from build123d import *

# Parameters (mm, degrees)
SKETCH1_R               = 4.765
BOSS_EXTRUDE2_DEPTH     = 9.5
CHAMFER1_SIZE           = 2.54
CHAMFER1_SIZE2          = 7.62
CHAMFER1_PART_2_SIZE    = 2.54
CHAMFER1_PART_2_SIZE2   = 7.62
CHAMFER2_SIZE           = 7.62
CHAMFER2_SIZE2          = 2.54
SKETCH3_W               = 9.53
SKETCH3_H               = 9.53
CUT_EXTRUDE1_DEPTH      = 20.54
CUT_EXTRUDE2_DEPTH      = 10.77
CUT_EXTRUDE2_DEPTH_BACK = 10.77
SKETCH5_R               = 1.59
CUT_EXTRUDE3_DEPTH      = 10.5000001
CUT_EXTRUDE3_DEPTH_BACK = 10.5000001


with BuildPart() as part:
    # Sketch1 → Boss-Extrude2 (new body, symmetric)
    with BuildSketch(Plane.XY):
        with BuildLine():
            Line((0, 9.77), (-22.23, 9.77))
            Line((-22.23, 9.77), (-22.23, 4.77))
            Line((-22.23, 4.77), (-9.711509246, -1.067468107))
            ThreePointArc((-9.711509246, -1.067468107), (-6.021421721, -7.693853421), (1.29754109, -9.683454297))
            Line((1.29754109, -9.683454297), (28.58, -6.027722532))
            Line((28.58, -6.027722532), (28.58, 0))
            Line((28.58, 0), (9.77, 0))
            ThreePointArc((9.77, 0), (6.908433252, 6.908433252), (0, 9.77))
        make_face()
        Circle(SKETCH1_R, mode=Mode.SUBTRACT)
    extrude(amount=BOSS_EXTRUDE2_DEPTH, both=True)

    # Chamfer1
    chamfer1_edges = [part.edges().sort_by_distance(p)[0] for p in [
        (-22.23, 7.27, 9.5),
    ]]
    chamfer1_side = [part.faces().sort_by_distance(p)[0] for p in [
        (-22.23, 7.27, 0),
    ]]
    chamfer(chamfer1_edges, length=CHAMFER1_SIZE, length2=CHAMFER1_SIZE2, reference=chamfer1_side[0])

    # Chamfer1 part 2
    chamfer1_part_2_edges = [part.edges().sort_by_distance(p)[0] for p in [
        (28.58, -3.013861266, 9.5),
    ]]
    chamfer1_part_2_side = [part.faces().sort_by_distance(p)[0] for p in [
        (28.58, -3.013861266, 0),
    ]]
    chamfer(chamfer1_part_2_edges, length=CHAMFER1_PART_2_SIZE, length2=CHAMFER1_PART_2_SIZE2, reference=chamfer1_part_2_side[0])

    # Chamfer2
    chamfer2_edges = [part.edges().sort_by_distance(p)[0] for p in [
        (-22.23, 7.27, -9.5),
        (28.58, -3.013861266, -9.5),
    ]]
    chamfer2_side = [part.faces().sort_by_distance(p)[0] for p in [
        (-11.115, 9.225622585, -9.5),
    ]]
    chamfer(chamfer2_edges, length=CHAMFER2_SIZE, length2=CHAMFER2_SIZE2, reference=chamfer2_side[0])

    # Sketch3 → Cut-Extrude1 (cut, through all)
    with BuildSketch(Plane(origin=(0, 9.77, 0), x_dir=(1, 0, 0), z_dir=(0, 1, 0))):
        with Locations((-17.465, 0)):
            Rectangle(SKETCH3_W, SKETCH3_H)
        with Locations((23.815, 0)):
            Rectangle(SKETCH3_W, SKETCH3_H)
    extrude(amount=-CUT_EXTRUDE1_DEPTH, mode=Mode.SUBTRACT)

    # Sketch4 → Cut-Extrude2 (cut, two sides)
    with BuildSketch(Plane(origin=(0, 0, 0), x_dir=(1, 0, 0), z_dir=(0, 1, 0))) as cut_extrude2_sk:
        with BuildLine():
            Line((-3.81, 5.08), (6.35, 5.08))
            ThreePointArc((6.35, 5.08), (11.43, 0), (6.35, -5.08))
            Line((6.35, -5.08), (-3.81, -5.08))
            ThreePointArc((-3.81, -5.08), (-8.89, 0), (-3.81, 5.08))
        make_face()
    extrude(amount=CUT_EXTRUDE2_DEPTH, mode=Mode.SUBTRACT)
    extrude(cut_extrude2_sk.sketch, amount=-CUT_EXTRUDE2_DEPTH_BACK, mode=Mode.SUBTRACT)

    # Sketch5 → Cut-Extrude3 (cut, two sides)
    with BuildSketch(Plane.XY) as cut_extrude3_sk:
        with Locations((-19.69, 7.23)):
            Circle(SKETCH5_R)
        with Locations((26.04, -2.54)):
            Circle(SKETCH5_R)
    extrude(amount=CUT_EXTRUDE3_DEPTH, mode=Mode.SUBTRACT)
    extrude(cut_extrude3_sk.sketch, amount=-CUT_EXTRUDE3_DEPTH_BACK, mode=Mode.SUBTRACT)


solid = part.part
Part model, mm, in its own coordinate system. A direction names the side the tool comes from. Coordinates: 2 decimals unless noted, no trailing zeros. Write each loop counter-clockwise with the first axis right and the second up, starting at its lowest first coordinate (ties: lowest second). Pieces come first, ordered by that corner, then holes. Notation, with made-up numbers: (24, 27.25) - (57, 27.25) arc R10 ccw to (57, 40.25) - close; hole circle Ø2 at (-21.75, -17). An arc over 180 degrees is marked (long way). Put each result on its own line as item: value.
1. Two-plate mould, pull along X, no slides. Class faces 1 (the flat face through (3, 4, -9.5)), 2 (the cylindrical face through (24.45, -2.47, -6.15)), 3 (the cylindrical face through (6.984, 6.832, -7.226)): +X half, -X half, draft (parallel to the pull), parting line (faces both ways), or undercut.
Final values:
face 1: draft
face 2: undercut
face 3: +X half
2. Band-saw the part on A-A (z = 6). Write the cut outline in (x, y) (1 decimal).
Final values:
outline: (-22.2, 4.8) - (-9.7, -1.1) arc R9.8 ccw to (1.3, -9.7) - (28.6, -6) - (28.6, 0) - (9.8, 0) arc R9.8 ccw to (0, 9.8) - (-22.2, 9.8) - close; hole circle Ø3.2 at (-19.7, 7.2); hole circle Ø9.5 at (0, 0); hole circle Ø3.2 at (26, -2.5)
3. Flat gauge pins, fed straight in: pin 1 Ø5 at (x, y) = (-19.69, 7.23) entering from -Z; pin 2 Ø4.5 at (x, y) = (-18, 5.5) entering from -Z; pin 3 Ø2 at (y, z) = (-3, -1) entering from +X. Where does each tip first touch, or does it go through?
Final values:
pin 1: stops at z = -8.64
pin 2: stops at z = -9.12
pin 3: stops at x = 19.05
4. Band-saw the part on D-D (z = 0). Write the cut outline in (x, y), then the cut area to 3 significant figures.
Final values:
outline: (-12.7, 0.33) - (-9.71, -1.07) arc R9.77 ccw to (-8.89, -4.05) - (-8.89, 9.77) - (-12.7, 9.77) - close; (11.43, -8.33) - (19.05, -7.3) - (19.05, 0) - (11.43, 0) - close
area: 100 mm²
5. Probe line 1 along X through (y, z) = (-2.54, -5.55); line 2 along Z through (x, y) = (-14, 4) (3 decimals); line 3 along Z through (x, y) = (-17, 2.75) (3 decimals). List the from-to ranges inside material, lowest first. Write a range as [from, to].
Final values:
line 1: x = [-9.43, -4.03], [4.03, 24.45], [27.63, 28.58]
line 2: z = [-9.5, -4.765], [4.765, 9.5]
line 3: z = [-8.703, -4.765], [4.765, 8.703]
6. Band-saw the part on C-C (x = 26.04). Write the cut outline in (y, z) (3 decimals), then the cut area to 3 significant figures.
Final values:
outline: (-6.368, -7.807) - (-4.13, -7.807) - (-4.13, -4.765) - (-6.368, -4.765) - close; (-6.368, 4.765) - (-4.13, 4.765) - (-4.13, 7.807) - (-6.368, 7.807) - close; (-0.95, -7.807) - (0, -7.807) - (0, -4.765) - (-0.95, -4.765) - close; (-0.95, 4.765) - (0, 4.765) - (0, 7.807) - (-0.95, 7.807) - close
area: 19.4 mm²
7. 3-axis set-ups, long thin cutter, end or side, ignore diameter. For faces 4 (the flat face through (23.87, -3.57, 8.53)), 5 (the cylindrical face through (-8.89, 2.34, 0.11)), 6 (the flat face through (-16, 6, -4.765)): which of +Z, -Z, +X, -X, +Y, -Y reach the whole face in a straight line?
Final values:
face 4: +Z, +X, +Y, -Y
face 5: +Y, -Y
face 6: -X, +Y, -Y
8. Band-saw the part on B-B (x = -16). Write the cut outline in (y, z) (3 decimals).
Final values:
outline: (1.865, -9.037) - (9.77, -9.037) - (9.77, -4.765) - (1.865, -4.765) - close; (1.865, 4.765) - (9.77, 4.765) - (9.77, 9.037) - (1.865, 9.037) - close
